Read the model definition and answer for the solid it produces. Units are mm, in the model's axes. A direction names the side the tool comes from. Round coordinates to 2 decimals unless told otherwise and drop trailing zeros. Order: outer loops, then holes, each group sorted by start corner. A loop starts at its lowest first (then second) coordinate and runs counter-clockwise, first axis right, second up.
from build123d import *

# Parameters (mm, degrees)
F0_W     = 76.2
F0_H     = 50.8
F1_DEPTH = 63.5
F2_W     = 12.7
F2_H     = 50.8
F3_DEPTH = 25.4
F4_W     = 25.4
F4_H     = 25.4
F5_DEPTH = 25.4


with BuildPart() as f1:
    # F0 (on Front) → F1 (new body)
    with BuildSketch(Plane.XZ):
        with Locations((8.374921, 3.300743)):
            Rectangle(F0_W, F0_H)
    extrude(amount=F1_DEPTH)

    # F2 (on face) → F3 (cut)
    with BuildSketch(Plane.XY.offset(28.700743)):
        with Locations((-14.327138, -38.1)):
            Rectangle(F2_W, F2_H)
    extrude(amount=-F3_DEPTH, mode=Mode.SUBTRACT)

    # F4 (on face) → F5 (cut)
    with BuildSketch(Plane.XY.offset(28.700743)):
        with Locations((33.774921, -25.4)):
            Rectangle(F4_W, F4_H)
    extrude(amount=-F5_DEPTH, mode=Mode.SUBTRACT)


solid = f1.part
Q1. A cutting plane is placed at B-B, the plane x = 33. Give the vertices of the cut face in (y, z).
Outcome:
outline: (-63.5, -22.1) - (0, -22.1) - (0, 28.7) - (-12.7, 28.7) - (-12.7, 3.3) - (-38.1, 3.3) - (-38.1, 28.7) - (-63.5, 28.7) - close
Q2. For faces 1 (the face through (-20.677, -38, 16)), 2 (the face through (-29.725, -31, 3)), 3 (the face through (21.075, -26, 16)), determine the directions among +Z, -Z, +X, -X, +Y, -Y from which every point of the face is accessible in a straight line to the end or side of a thin tool.
Outcome:
face 1: +Z, -Y
face 2: +Z, -Z, -X, +Y, -Y
face 3: +Z, +X
Q3. A cutting plane is placed at C-C, the plane z = 10. Give the vertices of the cut face in (x, y), plus the area to 3 significant figures.
Outcome:
outline: (-29.73, -63.5) - (-20.68, -63.5) - (-20.68, -12.7) - (-7.98, -12.7) - (-7.98, -63.5) - (46.47, -63.5) - (46.47, -38.1) - (21.07, -38.1) - (21.07, -12.7) - (46.47, -12.7) - (46.47, 0) - (-29.73, 0) - close
area: 3,550 mm2
Q4. Straight lines are drawn through the part: probe 1 along Y at (x, z) = (22.5, 5.5); probe 2 along X at (y, z) = (-38, 24); probe 3 along Z at (x, y) = (-17, -39). For each, find the intervals that lie inside material, in ascending order.
Outcome:
probe 1: y = -63.5 to -38.1, -12.7 to 0
probe 2: x = -29.73 to -20.68, -7.98 to 21.07
probe 3: z = -22.1 to 3.3
Q5. A cutting plane is placed at D-D, the plane y = -16.5. Give the vertices of the cut face in (x, z), plus the area to 3 significant figures.
Outcome:
outline: (-29.73, -22.1) - (46.47, -22.1) - (46.47, 3.3) - (21.07, 3.3) - (21.07, 28.7) - (-7.98, 28.7) - (-7.98, 3.3) - (-20.68, 3.3) - (-20.68, 28.7) - (-29.73, 28.7) - close
area: 2,900 mm2
Q6. A cutting plane is placed at A-A, the plane y = -53. Give the vertices of the cut face in (x, z), plus the area to 3 significant figures.
Outcome:
outline: (-29.73, -22.1) - (46.47, -22.1) - (46.47, 28.7) - (-7.98, 28.7) - (-7.98, 3.3) - (-20.68, 3.3) - (-20.68, 28.7) - (-29.73, 28.7) - close
area: 3,550 mm2
Q7. For a pull along Y with two mould halves and no side action, classify faces 4 (the face through (-14, -12.7, 16)), 5 (the face through (8, -31, -22.099)), 6 (the face through (34, -38.1, 16)) as released by +Y, released by -Y, zero draft, split by the parting line, or undercut.
Outcome:
face 4: released by -Y
face 5: zero draft
face 6: undercut
Q8. Flat-ended cylindrical pins translate along their axes: pin 1 (10 mm diameter, centred on x = -15, z = 12.5, fed in from -Y); pin 2 (20.5 mm diameter, centred on y = -24.5, z = 19, fed in from +X); pin 3 (6.5 mm diameter, centred on x = -11.5, y = -31, fed in from +Z). Find the tip coordinate at first contact, or state that the pin passes through.
Outcome:
pin 1: stops at y = -12.7
pin 2: stops at x = 21.07
pin 3: stops at z = 3.3
